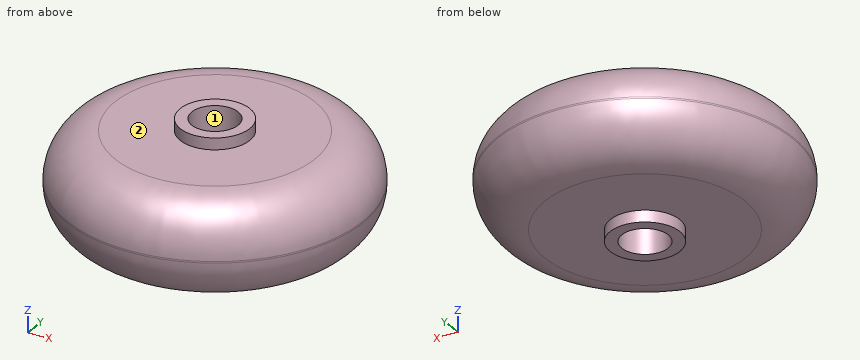
from build123d import *

# Parameters (mm, degrees)
ESQUISSE1_R             = 25.4
ESQUISSE1_R_2           = 4
BOSS_EXTRU_1_DEPTH      = 16.66
BOSS_EXTRU_2_DEPTH      = 2
BOSS_EXTRU_2_DEPTH_BACK = 18.66
ESQUISSE2_R             = 6
ESQUISSE2_R_2           = 4
CONG_1_R                = 8.2


with BuildPart() as part:
    # Esquisse1 → Boss.-Extru.1 (new body)
    with BuildSketch(Plane.XY):
        Circle(ESQUISSE1_R)
        Circle(ESQUISSE1_R_2, mode=Mode.SUBTRACT)
    extrude(amount=BOSS_EXTRU_1_DEPTH)

    # Esquisse2 → Boss.-Extru.2 (add, two sides: drawn at the far end of the back side and taken through both)
    with BuildSketch(Plane.XY.offset(16.66).offset(-BOSS_EXTRU_2_DEPTH_BACK)):
        Circle(ESQUISSE2_R)
        Circle(ESQUISSE2_R_2, mode=Mode.SUBTRACT)
    extrude(amount=BOSS_EXTRU_2_DEPTH + BOSS_EXTRU_2_DEPTH_BACK)

    # Congé1
    cong_1_edges = [part.edges().sort_by_distance(p)[0] for p in [
        (-25.4, 0, 0),
        (-25.4, 0, 16.66),
    ]]
    fillet(cong_1_edges, radius=CONG_1_R)


solid = part.part
Design review of the part built by this model. Coordinates are the model's own, in mm. Face numbers are marked on the shaded views. Round coordinates to 2 decimals unless told otherwise and drop trailing zeros. Order: outer loops, then holes, each group sorted by start corner. A loop starts at its lowest first (then second) coordinate and runs counter-clockwise, first axis right, second up. Notation, with made-up numbers: M -8,31 L 46,31 A16 cw 46,37 Z; hole C 7.5,84 d10. An arc over 180 degrees is marked long. Answer as CSV lines item,"result". Start each with the question number.
1) For pin 1 Ø17 at (x, y) = (2, -3) entering from -Z; pin 2 Ø2 at (x, y) = (-0.5, 2.5) entering from +Z; pin 3 Ø4 at (x, y) = (-5.5, -10) entering from +Z; pin 4 Ø1.5 at (x, z) = (4.5, 2.5) entering from -Y, all flat-tipped, find the tip position at first contact; note any pin that passes through.
2) Add section A-A (x = 0). Give the boundary of the cut face in (y, z).
3) Add section D-D (z = 0.75). Give the boundary of the cut face in (x, y), then the cut area to 3 significant figures.
4) Add section C-C (z = 13). Give the boundary of the cut face in (x, y).
5) The part is to be moulded in two halves that separate along Y. For the marked faces 1 and 2, say which applies: +Y half, -Y half, draft (parallel to the pull), parting line (faces both ways), or undercut.
6) Wall thickness on line 1 along Y through (x, z) = (-1, 2); line 2 along Y through (x, z) = (0, 6); line 3 along Z through (x, y) = (-11.5, -7.5): over which ranges is each line inside the solid? List them lowest first. Write a range as [from, to].
Resolved:
1,pin 1,"z = -2"
1,pin 2,"through"
1,pin 3,"z = 16.66"
1,pin 4,"y = -23.32"
2,outline,"M -25.4,8.2 A8.2 ccw -17.2,0 L -6,0 L -6,-2 L -4,-2 L -4,18.66 L -6,18.66 L -6,16.66 L -17.2,16.66 A8.2 ccw -25.4,8.46 Z; M 4,-2 L 6,-2 L 6,0 L 17.2,0 A8.2 ccw 25.4,8.2 L 25.4,8.46 A8.2 ccw 17.2,16.66 L 6,16.66 L 6,18.66 L 4,18.66 Z"
3,outline,"C 0,0 d41.25; hole C 0,0 d8"
3,area,"1,290 mm^2"
4,outline,"C 0,0 d48.06; hole C 0,0 d8"
5,face 1,"undercut"
5,face 2,"draft"
6,line 1,"[-22.54, -3.87], [3.87, 22.54]"
6,line 2,"[-25.1, -4], [4, 25.1]"
6,line 3,"[0, 16.66]"
